```python
from build123d import *

# Parameters (mm, degrees)
SKETCH1_R           = 1.5
SKETCH1_R_2         = 11
SKETCH1_R_3         = 1.65
BOSS_EXTRUDE1_DEPTH = 5
FILLET1_R           = 10
FILLET2_R           = 5


with BuildPart() as part:
    # Sketch1 → Boss-Extrude1 (new body)
    with BuildSketch(Plane.XY):
        Polygon((23.883435073, 30), (43.883435073, 30), (43.883435073, -45), (-5.116564927, -45), (-5.116564927, 0), (0, 0), (23.883435073, 0), align=None)
        with Locations((3.883435073, -5)):
            Circle(SKETCH1_R, mode=Mode.SUBTRACT)
        with Locations((34.883435073, -5)):
            Circle(SKETCH1_R, mode=Mode.SUBTRACT)
        with Locations((3.883435073, -36)):
            Circle(SKETCH1_R, mode=Mode.SUBTRACT)
        with Locations((34.883435073, -36)):
            Circle(SKETCH1_R, mode=Mode.SUBTRACT)
        with Locations((19.383435073, -20.5)):
            Circle(SKETCH1_R_2, mode=Mode.SUBTRACT)
        with Locations((33.883435073, 15)):
            Circle(SKETCH1_R_3, mode=Mode.SUBTRACT)
    extrude(amount=BOSS_EXTRUDE1_DEPTH)

    # Fillet1
    fillet1_edges = [part.edges().sort_by_distance(p)[0] for p in [
        (23.883435073, 0, 2.5),
        (43.883435073, -45, 2.5),
        (-5.116564927, -45, 2.5),
        (-5.116564927, 0, 2.5),
    ]]
    fillet(fillet1_edges, radius=FILLET1_R)

    # Fillet2
    fillet2_edges = [part.edges().sort_by_distance(p)[0] for p in [
        (23.883435073, 30, 2.5),
        (43.883435073, 30, 2.5),
    ]]
    fillet(fillet2_edges, radius=FILLET2_R)


solid = part.part
```
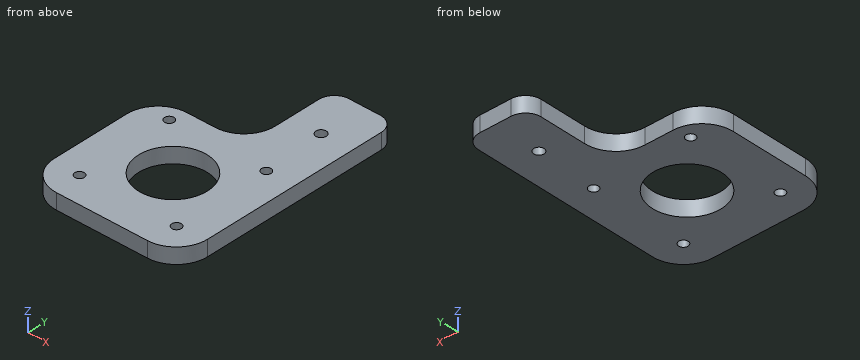
Here's how the part is built. I have some questions about the finished solid (model axes, mm). Coordinates: 2 decimals unless noted, no trailing zeros. Loops run counter-clockwise (first coordinate to the right, second up) from the corner with the lowest first, then second, coordinate; pieces in that order, holes last. Notation, with made-up numbers: (-22.75, -23) -> (23.25, -23) arc R26 cw to (23.25, 8) -> close; hole circle Ø11 at (47.25, 63.25). An arc over 180 degrees is marked (long way). Return JSON: item names as keys, results as strings.
1) I need wall thicknesses on line 1 (X direction, y = 23.5, z = 3.15); line 2 (Y direction, x = 22.5, z = 4.3); line 3 (Y direction, x = 15.5, z = 3.1). Which ranges of each line are inside material? Lowest first, please. Write a range as from..to.
Results below:
{"line 1": "23.88..43.88", "line 2": "-45..-31.05, -9.95..4.93", "line 3": "-45..-30.79, -10.21..0.13"}
2) If we section it at C-C, the plane x = 17.5: Write out the boundary of the cut face in (y, z).
Results below:
{"outline": "(-45, 0) -> (-31.34, 0) -> (-31.34, 5) -> (-45, 5) -> close; (-9.66, 0) -> (0.68, 0) -> (0.68, 5) -> (-9.66, 5) -> close"}
3) If we section it at D-D, the plane y = -36: Write out the boundary of the cut face in (x, z), then the cut area to 3 significant figures.
Results below:
{"outline": "(-5.07, 0) -> (2.38, 0) -> (2.38, 5) -> (-5.07, 5) -> close; (5.38, 0) -> (33.38, 0) -> (33.38, 5) -> (5.38, 5) -> close; (36.38, 0) -> (43.83, 0) -> (43.83, 5) -> (36.38, 5) -> close", "area": "214 mm²"}
4) Will this pin go through, and if not, where does the flat tip stop? pin 1 (13 mm diameter, centred on x = 19.38, y = -20.5, fed in from +Z).
Results below:
{"pin 1": "through"}
5) If we section it at A-A, the plane z = 2.7: Write out the boundary of the cut face in (x, y), then the cut area to 3 significant figures.
Results below:
{"outline": "(-5.12, -35) arc R10 ccw to (4.88, -45) -> (33.88, -45) arc R10 ccw to (43.88, -35) -> (43.88, 25) arc R5 ccw to (38.88, 30) -> (28.88, 30) arc R5 ccw to (23.88, 25) -> (23.88, 10) arc R10 cw to (13.88, 0) -> (4.88, 0) arc R10 ccw to (-5.12, -10) -> close; hole circle Ø3 at (3.88, -36); hole circle Ø3 at (3.88, -5); hole circle Ø22 at (19.38, -20.5); hole circle Ø3.3 at (33.88, 15); hole circle Ø3 at (34.88, -36); hole circle Ø3 at (34.88, -5)", "area": "2,330 mm²"}
6) If we section it at B-B, the plane y = 15: Write out the boundary of the cut face in (x, z), then the cut area to 3 significant figures.
Results below:
{"outline": "(23.88, 0) -> (32.23, 0) -> (32.23, 5) -> (23.88, 5) -> close; (35.53, 0) -> (43.88, 0) -> (43.88, 5) -> (35.53, 5) -> close", "area": "83.5 mm²"}
